Study the drawing (mm; zero at the part's minimum x, y, z) and answer. A direction names the side the tool comes from. Coordinates: 2 decimals unless noted, no trailing zeros. Order: outer loops, then holes, each group sorted by start corner. A loop starts at its lowest first (then second) coordinate and runs counter-clockwise, first axis right, second up. Notation, with made-up numbers: (0.5, 67.5) - (42.5, 67.5) arc R28 cw to (42.5, 89.5) - close; hole circle Ø5 at (-20, 66). An arc over 180 degrees is marked (long way). Write item = value, one per line.
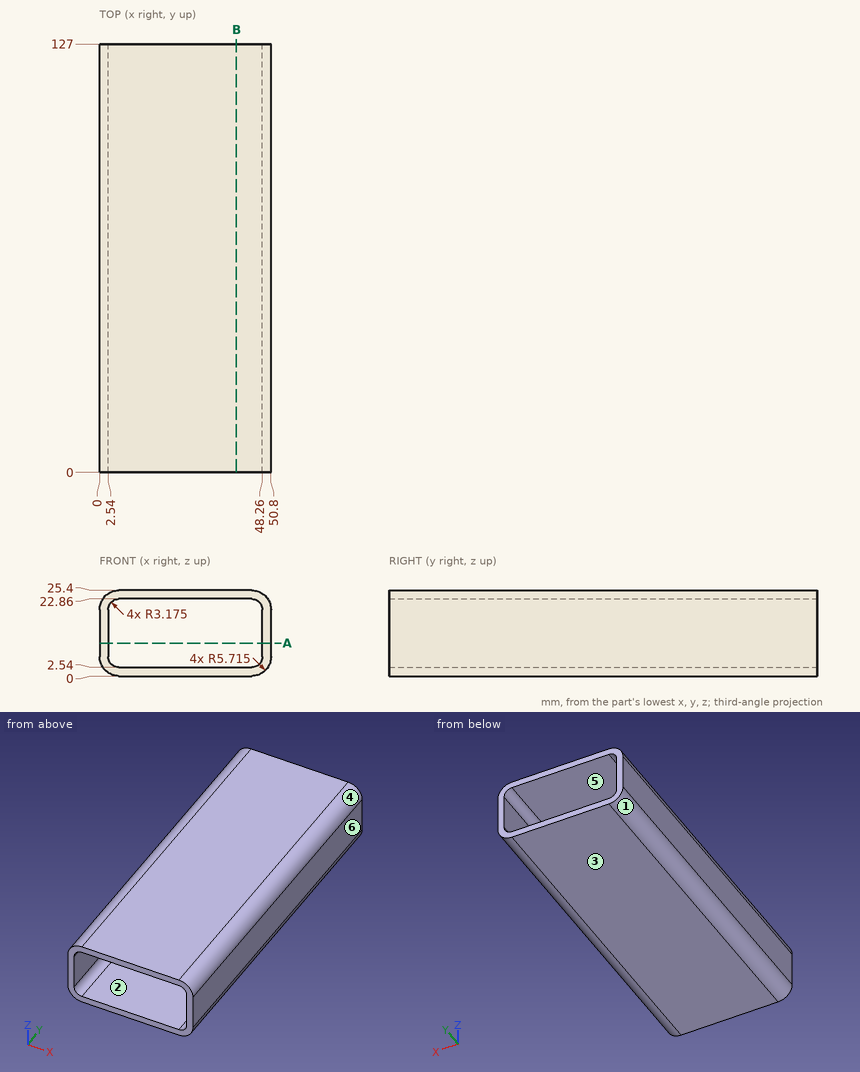
1) The part is cut by section B-B (x = 40.5). Determine the outline of the cut face in (y, z), and give its area (3 significant figures).
Returned:
outline = (0, 0) - (127, 0) - (127, 2.54) - (0, 2.54) - close; (0, 22.86) - (127, 22.86) - (127, 25.4) - (0, 25.4) - close
area = 645 mm^2
2) The part is cut by section A-A (z = 9.75). Determine the outline of the cut face in (x, y).
Returned:
outline = (0, 0) - (2.54, 0) - (2.54, 127) - (0, 127) - close; (48.26, 0) - (50.8, 0) - (50.8, 127) - (48.26, 127) - close
3) Straight lines are drawn through the part: line 1 along X through (y, z) = (91, 19); line 2 along Z through (x, y) = (44.5, 20.5); line 3 along X through (y, z) = (75, 3.5) (1 decimal). For each, find the intervals that lie inside material, in ascending order. Write a range as from..to.
Returned:
line_1 = 0..2.54, 48.26..50.8
line_2 = 0..2.54, 22.86..25.4
line_3 = 0.4..3.4, 47.4..50.4
4) For the marked faces 1 and 2, determine the directions among +Z, -Z, +X, -X, +Y, -Y from which every point of the face is accessible in a straight line to the end or side of a thin tool.
Returned:
face_1 = -Z, -X, +Y, -Y
face_2 = +Y, -Y
5) A flat-ended cylindrical pin translates along its axis: pin 1 Ø3 at (y, z) = (48.5, 22) entering from +X. Find the tip coordinate at first contact, or state that the pin passes through.
Returned:
pin_1 = 50.74
6) Determine the mould class of the marked faces 3, 4, 5 and 6 for opening direction Z: pulls with the +Z half, pulls with the -Z half, needs draft (parallel to the pull), parting line crosses it, or undercut.
Returned:
face_3 = pulls with the -Z half
face_4 = pulls with the +Z half
face_5 = undercut
face_6 = needs draft
